from build123d import *

# Parameters (mm, degrees)
RESSALTO_EXTRUS_O1_DEPTH                       = 2
BROCA_DE_ROSQUEAR_DE_CANO_PARA_TARRAXA_D_D     = 6
BROCA_DE_ROSQUEAR_DE_CANO_PARA_TARRAXA_D_DEPTH = 4
BROCA_DE_ROSQUEAR_DE_CANO_PARA_TARRAXA_D_TIP   = 1.802581857


with BuildPart() as part:
    # Esboço1 → Ressalto-extrusão1 (new body)
    with BuildSketch(Plane(origin=(0, 0, 0), x_dir=(0, 0, -1), z_dir=(1, 0, 0))):
        Polygon((-131, -26), (-131, -37.5), (187, -37.5), (187, 34.5), align=None)
    extrude(amount=RESSALTO_EXTRUS_O1_DEPTH)

    # Broca de rosquear de cano para tarraxa de 1/810
    with Locations(Plane(origin=(2, 0, 0), x_dir=(0, 0, -1), z_dir=(1, 0, 0))):
        with Locations((-105.202549234, -31.420254628)):
            Hole(BROCA_DE_ROSQUEAR_DE_CANO_PARA_TARRAXA_D_D / 2, depth=BROCA_DE_ROSQUEAR_DE_CANO_PARA_TARRAXA_D_DEPTH)
            with Locations((0, 0, -(BROCA_DE_ROSQUEAR_DE_CANO_PARA_TARRAXA_D_DEPTH + BROCA_DE_ROSQUEAR_DE_CANO_PARA_TARRAXA_D_TIP / 2))):  # 118° drill point
                Cone(0, BROCA_DE_ROSQUEAR_DE_CANO_PARA_TARRAXA_D_D / 2, BROCA_DE_ROSQUEAR_DE_CANO_PARA_TARRAXA_D_TIP, mode=Mode.SUBTRACT)


solid = part.part
Design review of the part built by this model. Coordinates are the model's own, in mm. Round coordinates to 2 decimals unless told otherwise and drop trailing zeros. Loops run counter-clockwise (first coordinate to the right, second up) from the corner with the lowest first, then second, coordinate; pieces in that order, holes last. Notation, with made-up numbers: (4, -31.75) - (12, -31.75) arc R10 cw to (12, -18.75) - close; hole circle Ø3 at (-10.5, 39.5). An arc over 180 degrees is marked (long way). One line per item, written item: value. Start each with the question number.
1) Consider section B-B on z = 36.5. Give the boundary of the cut face in (x, y), then the cut area to 3 significant figures.
2) Consider section A-A on x = 1.55. Give the boundary of the cut face in (y, z).
3) To check wall thickness, follow L1, parallel to Z at x = 1.85, y = -29; L2, parallel to Y at x = 1.2, z = -82.5; L3, parallel to Y at x = 1.55, z = -124. State the ranges of each line that lie inside material, in increasing order. Write a range as from..to.
4) Draft analysis for pull direction Y (two halves, no side actions). For faces 1 (the flat face through (0.986, 4.673, -30.226)), 2 (the cylindrical face through (0.986, -31.288, 102.205)), 3 (the flat face through (2, -9, -61)), state which applies: +Y half, -Y half, draft (parallel to the pull), parting line (faces both ways), or undercut.
5) Consider section C-C on y = 3.5. Give the boundary of the cut face in (x, z).
Reported:
1. outline: (0, -37.5) - (2, -37.5) - (2, -8.02) - (0, -8.02) - close
1. area: 59.0 mm^2
2. outline: (-37.5, -187) - (34.5, -187) - (-26, 131) - (-37.5, 131) - close; hole circle Ø6 at (-31.42, 105.2)
3. L1: z = -187..103.43, 106.98..131
3. L2: y = -37.5..14.62
3. L3: y = -37.5..22.51
4. face 1: +Y half
4. face 2: undercut
4. face 3: draft
5. outline: (0, -187) - (2, -187) - (2, -24.06) - (0, -24.06) - close
